Autodesk Inventor part; units mm, degrees
ref_plane "YZ Plane" through (0, 0, 0) normal (1, 0, 0) x (0, 1, 0)
ref_plane "XZ Plane" through (0, 0, 0) normal (0, 1, 0) x (-1, 0, 0)
ref_plane "XY Plane" through (0, 0, 0) normal (0, 0, 1) x (1, 0, 0)
sketch "Sketch1" plane through (0, 0, 0) normal (0, 1, 0) x (-1, 0, 0)
  circle A0 centre (0, 0) radius 50
  line L0 (35.3554, -35.3553) -> (42.8554, -35.3553) construction
  line L1 (48.2963, -12.941) -> (55.7963, -12.941) construction
  line L2 (12.9409, 48.2963) -> (20.4409, 48.2963) construction
  line L3 (-12.941, 48.2963) -> (-5.441, 48.2963) construction
  line L4 (-48.2963, -12.941) -> (-40.7963, -12.941) construction
  line L5 (-35.3553, -35.3553) -> (-27.8553, -35.3553) construction
  line L6 (45.3554, -35.3553) -> (53.2963, -21.6012)
  line L7 (-45.3554, -35.3553) -> (-53.2964, -21.6012)
  line L8 (-7.941, 56.9566) -> (7.9409, 56.9566)
  line L9 (7.9409, 56.9566) -> (53.2963, -21.6012)
  line L10 (-45.3554, -35.3553) -> (45.3554, -35.3553)
  line L11 (-53.2964, -21.6012) -> (-7.941, 56.9566)
  line L12 (44.636, -21.6012) -> (41.0252, -27.8553)
  line L13 (41.0252, -27.8553) -> (-41.0253, -27.8553)
  line L14 (-41.0253, -27.8553) -> (-44.6361, -21.6012)
  line L15 (-44.6361, -21.6012) -> (-3.6108, 49.4566)
  line L16 (-3.6108, 49.4566) -> (3.6108, 49.4566)
  line L17 (3.6108, 49.4566) -> (44.636, -21.6012)
  arc A1 (0, -27.8553) -> (0.0657, -27.8553) centre (0.0328, 0.0001) ccw
  circle A2 centre (0, 0) radius 22.5
  line L18 (3.6108, -27.8553) -> (-3.6108, -27.8553)
  line L19 (-3.6108, -27.8553) -> (-3.6108, 49.4566)
  line L20 (-3.6108, 49.4566) -> (3.6108, 49.4566)
  line L21 (3.6108, 49.4566) -> (3.6108, -27.8553)
  circle A3 centre (0, 0) radius 30
  point P0 (0, -27.8553)
  point P1 (0, -27.8553)
  point P2 (0, 49.4566)
  point P3 (0, 49.4566)
  dimension "d0" = 100
  dimension "d7" = 35.3553
  dimension "d9" = 12.941
  dimension "d10" = 48.2963
  dimension "d11" = 35.3553
  dimension "d12" = 35.3553
  dimension "d13" = 35.3554
  dimension "d17" = 12.941
  dimension "d18" = 48.2963
  dimension "d20" = 48.2963
  dimension "d21" = 12.9409
  dimension "d22" = 48.2963
  dimension "d23" = 12.941
  dimension "d99" = 7.5
  dimension "d133" = 2.5
  dimension "d134" = 15.8819
  dimension "d140" = 15.8819
  dimension "d143" = 15.8819
  dimension "d144" = 90.7107
  dimension "d145" = 90.7108
  dimension "d146" = 90.7107
  dimension "d147" = 35.3553
  dimension "d148" = 120
  dimension "d149" = 120
  dimension "d150" = 7.5
  dimension "d184" = 45
  dimension "d185" = 60
extrude "Extrusion5" add sketch "Sketch1" along normal blind 13 contours L9 A0 L10 L11 | A0 L11 L8 L9 | L9 L6 L10 A0 | A0 L10 L7 L11 | L17 A3 | A3 L13 | A3 L15
sketch "Sketch5" plane through (53.2964, 0, -21.6012) normal (0.866, 0, 0.5) x (0.5, 0, -0.866)
  circle A0 centre (-80.7107, 9) radius 2
  circle A1 centre (-10, 9) radius 2
  line L0 (-90.7107, 13) -> (0, 13)
  line L1 (-90.7107, 0) -> (-90.7107, 13)
  line L2 (0, 0) -> (0, 13)
  point P0 (-45.3554, 0)
  dimension "d155" = 4
  dimension "d156" = 4
  dimension "d157" = 4
  dimension "d158" = 10
  dimension "d159" = 10
sketch "Sketch6" plane through (-7.9409, 0, 56.9566) normal (-0.866, 0, 0.5) x (0.5, 0, 0.866)
  circle A0 centre (-80.7107, 9) radius 2
  circle A1 centre (-10, 9) radius 2
  line L0 (0, 0) -> (0, 13)
  line L1 (-90.7107, 13) -> (0, 13)
  line L2 (-90.7107, 0) -> (-90.7107, 13)
  point P0 (-45.3554, 0)
  dimension "d160" = 4
  dimension "d161" = 4
  dimension "d162" = 10
  dimension "d163" = 4
  dimension "d164" = 10
sketch "Sketch7" plane through (45.3554, 0, -35.3553) normal (0, 0, -1) x (-1, 0, 0)
  circle A0 centre (10, 9) radius 2
  circle A1 centre (80.7107, 9) radius 2
  line L0 (0, 13) -> (90.7107, 13)
  line L1 (0, 0) -> (0, 13)
  line L2 (90.7107, 0) -> (90.7107, 13)
  point P0 (45.3554, 0)
  dimension "d165" = 4
  dimension "d166" = 4
  dimension "d167" = 4
  dimension "d168" = 10
  dimension "d169" = 10
extrude "Extrusion6" cut sketch "Sketch5" against normal blind 7.5
extrude "Extrusion7" cut sketch "Sketch7" against normal blind 7.5
extrude "Extrusion8" cut sketch "Sketch6" against normal blind 7.5
extrude "Extrusion9" add sketch "Sketch1" along normal blind 3 contours A3 L13 L21 A2 L17 | L17 A3 | A3 L13 | L13 L19 A2 L21 | A3 L15 L19 A2 L13 | L21 A3 L19 L16 | L21 A2 L19 A3 | A2 L19 L21 | A3 L15
properties part number "Stewart_Platform"
Part model, mm, in its own coordinate system. A direction names the side the tool comes from. Coordinates: 2 decimals unless noted, no trailing zeros. Write each loop counter-clockwise with the first axis right and the second up, starting at its lowest first coordinate (ties: lowest second). Pieces come first, ordered by that corner, then holes.
Item 1: Probe line 1 (Z direction, x = 14, y = 1); line 2 (Z direction, x = -10, y = 10.5); line 3 (Y direction, x = 1, z = -25.5). List the from-to ranges inside material, lowest first.
Item 2: Slice it at A-A (y = 5.75). Write the cut outline in (x, z), and give its area (3 significant figures).
Item 3: Slice it at B-B (z = -3.5). Write the cut outline in (x, y), and give its area (3 significant figures).
Item 4: Pin check, flat tips, straight feed: pin 1 (3.5 mm diameter, centred on y = 1, z = 36.5, fed in from +X); pin 2 (6 mm diameter, centred on y = 10, z = 17, fed in from -X); pin 3 (6.5 mm diameter, centred on x = 17.5, y = 5, fed in from +Z). Stop position of each tip, or through.
Item 5: Mould opens along Z. For faces 4 (the face through (-33.88, 10.35, -31.66)), 5 (the face through (0, 6, 56.957)), 6 (the face through (-42.86, 6.41, -24.68)) say: released by +Z, released by -Z, zero draft, split by the parting line, or undercut.
Item 6: Slice it at C-C (z = 34). Write the cut outline in (x, y) (3 decimals).
Item 7: Which spindle directions (+Z, -Z, +X, -X, +Y, -Y) get a long thin tool onto all of the face, cutting with end or side? Do faces 1 (the face through (37.353, 9.088, -31.658)), 2 (the face through (-3.611, 1, 40)), 3 (the face through (0, 8, 49.457)). Say none if no direction does.
Results found:
1. line 1: z = -35.36 to -27.86, -26.53 to -17.61, 17.61 to 26.53, 31.46 to 46.46
1. line 2: z = -35.36 to -27.86, 38.39 to 45.07, 48.13 to 53.39
1. line 3: y = 0 to 3
2. outline: (-53.3, -21.6) - (-45.36, -35.36) - (45.36, -35.36) - (53.3, -21.6) - (7.94, 56.96) - (-7.94, 56.96) - close; hole (-44.64, -21.6) - (-41.03, -27.86) - (-0.07, -27.86) arc R27.94 ccw to (0, -27.86) - (41.03, -27.86) - (44.64, -21.6) - (3.61, 49.46) - (-3.61, 49.46) - close
2. area: 2,200 mm2
3. outline: (-42.85, 0) - (-34.19, 0) - (-34.19, 13) - (-42.85, 13) - close; (-29.8, 0) - (-22.23, 0) - (-22.23, 3) - (-29.8, 3) - close; (-3.61, 0) - (3.61, 0) - (3.61, 3) - (-3.61, 3) - close; (22.23, 0) - (29.8, 0) - (29.8, 3) - (22.23, 3) - close; (34.19, 0) - (42.85, 0) - (42.85, 13) - (34.19, 13) - close
3. area: 292 mm2
4. pin 1: stops at x = 20.76
4. pin 2: stops at x = -32.74
4. pin 3: stops at z = 46.03
5. face 4: zero draft
5. face 5: released by +Z
5. face 6: undercut
6. outline: (-21.195, 0) - (-12.535, 0) - (-12.535, 13) - (-21.195, 13) - close; (-3.611, 0) - (3.611, 0) - (3.611, 3) - (-3.611, 3) - close; (12.535, 0) - (21.195, 0) - (21.195, 13) - (12.535, 13) - close
7. face 1: -Z
7. face 2: +Y, -Y
7. face 3: +Y
